Geometry check sheet. Reference: the model listing, model coordinates, mm. Face numbers are marked on the shaded views. Round coordinates to 2 decimals unless told otherwise and drop trailing zeros. Order: outer loops, then holes, each group sorted by start corner. A loop starts at its lowest first (then second) coordinate and runs counter-clockwise, first axis right, second up.
(1) Sectioned sample at C-C (z = 3.15). Record the boundary of the cut face in (x, y), plus the area to 3 significant figures.
(2) Material ranges on line 1 along Y through (x, z) = (-103.5, 0.4); line 2 along X through (y, z) = (0.5, 1.1); line 3 along Y through (x, z) = (0, 3.35), recorded low to high.
(3) Sectioned sample at B-B (x = 0). Record the boundary of the cut face in (y, z), plus the area to 3 significant figures.
(4) Release check for a two-part mould opening along X. For the marked faces 1 and 2 record: +X half, -X half, draft (parallel to the pull), parting line (faces both ways), or undercut.
(5) Sectioned sample at D-D (y = 7). Give the number of separate pieces and of enclosed holes in the cut face, plus the area to 3 significant figures.
(6) Sectioned sample at A-A (x = -103.5). Record the boundary of the cut face in (y, z), plus the area to 3 significant figures.
(7) Go/stop test with flat-tipped pins: pin 1 (0.6 mm diameter, centred on x = 35, z = 0, fed in from +Y); pin 2 (3.5 mm diameter, centred on x = -103.5, y = 7, fed in from -Z); pin 3 (1 mm diameter, centred on y = -8, z = 1.5, fed in from +X); pin 4 (0.6 mm diameter, centred on x = 57.5, z = 0, fed in from -Y). Record where each tip stops, or that it passes through.
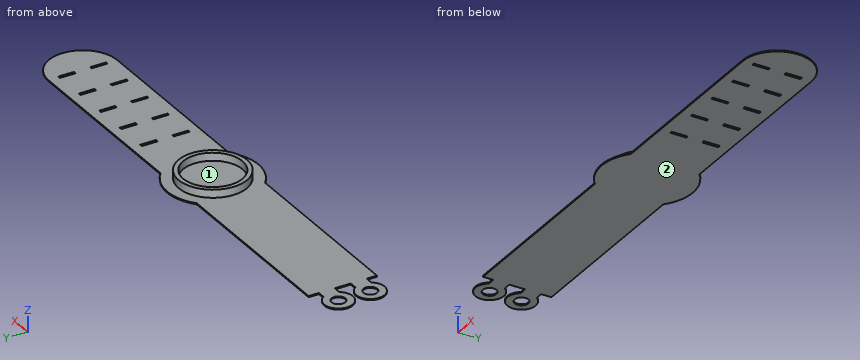
from build123d import *

# Parameters (mm, degrees)
SKETCH_1_W      = 1
SKETCH_1_H      = 7
SKETCH_1_W_2    = 1.2
SKETCH_1_R      = 3
EXTRUDE_2_DEPTH = 0.5
SKETCH_3_R      = 15
SKETCH_3_R_2    = 13
EXTRUDE_3_DEPTH = 4


with BuildPart() as part:
    # Эскиз1 → Бобышка-Вытянуть2 (new body)
    with BuildSketch(Plane.XY):
        with BuildLine():
            Line((95, 15), (13.228756555, 15))
            ThreePointArc((13.228756555, 15), (0, 20), (-13.228756555, 15))
            Line((-13.228756555, 15), (-95, 15))
            Line((-95, 15), (-95, 10.5))
            Line((-95, 10.5), (-98.321921206, 10.5))
            ThreePointArc((-98.321921206, 10.5), (-109.75, 7), (-98.321921206, 3.5))
            Line((-98.321921206, 3.5), (-95, 3.5))
            Line((-95, 3.5), (-95, -3.5))
            Line((-95, -3.5), (-98.321921206, -3.5))
            ThreePointArc((-98.321921206, -3.5), (-109.75, -7), (-98.321921206, -10.5))
            Line((-98.321921206, -10.5), (-95, -10.5))
            Line((-95, -10.5), (-95, -15))
            Line((-95, -15), (-13.228756555, -15))
            ThreePointArc((-13.228756555, -15), (0, -20), (13.228756555, -15))
            Line((13.228756555, -15), (95, -15))
            ThreePointArc((95, -15), (110, 0), (95, 15))
        make_face()
        with Locations((35, -7)):
            Rectangle(SKETCH_1_W, SKETCH_1_H, mode=Mode.SUBTRACT)
        with Locations((50, -7)):
            Rectangle(SKETCH_1_W, SKETCH_1_H, mode=Mode.SUBTRACT)
        with Locations((65, -7)):
            Rectangle(SKETCH_1_W, SKETCH_1_H, mode=Mode.SUBTRACT)
        with Locations((80, -7)):
            Rectangle(SKETCH_1_W, SKETCH_1_H, mode=Mode.SUBTRACT)
        with Locations((95, -7)):
            Rectangle(SKETCH_1_W, SKETCH_1_H, mode=Mode.SUBTRACT)
        with Locations((35, 7)):
            Rectangle(SKETCH_1_W_2, SKETCH_1_H, mode=Mode.SUBTRACT)
        with Locations((50, 7)):
            Rectangle(SKETCH_1_W_2, SKETCH_1_H, mode=Mode.SUBTRACT)
        with Locations((65, 7)):
            Rectangle(SKETCH_1_W_2, SKETCH_1_H, mode=Mode.SUBTRACT)
        with Locations((80, 7)):
            Rectangle(SKETCH_1_W_2, SKETCH_1_H, mode=Mode.SUBTRACT)
        with Locations((95, 7)):
            Rectangle(SKETCH_1_W_2, SKETCH_1_H, mode=Mode.SUBTRACT)
        with Locations((-103.5, 7)):
            Circle(SKETCH_1_R, mode=Mode.SUBTRACT)
        with Locations((-103.5, -7)):
            Circle(SKETCH_1_R, mode=Mode.SUBTRACT)
    extrude(amount=EXTRUDE_2_DEPTH)

    # Эскиз3 → Бобышка-Вытянуть3 (add)
    with BuildSketch(Plane(origin=(0, 0, 0), x_dir=(-1, 0, 0), z_dir=(0, 0, -1))):
        Circle(SKETCH_3_R)
        Circle(SKETCH_3_R_2, mode=Mode.SUBTRACT)
    extrude(amount=-EXTRUDE_3_DEPTH)


solid = part.part
Answer below:
1. outline: circle Ø30 at (0, 0); hole circle Ø26 at (0, 0)
1. area: 176 mm2
2. line 1: y = -13.25 to -10, -4 to -0.75, 0.75 to 4, 10 to 13.25
2. line 2: x = -14.99 to -12.99, 12.99 to 14.99
2. line 3: y = -15 to -13, 13 to 15
3. outline: (-20, 0) - (20, 0) - (20, 0.5) - (15, 0.5) - (15, 4) - (13, 4) - (13, 0.5) - (-13, 0.5) - (-13, 4) - (-15, 4) - (-15, 0.5) - (-20, 0.5) - close
3. area: 34.0 mm2
4. face 1: undercut
4. face 2: draft
5. separate pieces: 7
5. enclosed holes: 0
5. area: 119 mm2
6. outline: (-13.25, 0) - (-10, 0) - (-10, 0.5) - (-13.25, 0.5) - close; (-4, 0) - (-0.75, 0) - (-0.75, 0.5) - (-4, 0.5) - close; (0.75, 0) - (4, 0) - (4, 0.5) - (0.75, 0.5) - close; (10, 0) - (13.25, 0) - (13.25, 0.5) - (10, 0.5) - close
6. area: 6.50 mm2
7. pin 1: stops at y = 15
7. pin 2: passes through
7. pin 3: stops at x = 12.99
7. pin 4: stops at y = -15
